Read the model definition and answer for the solid it produces. Units are mm, in the model's axes. A direction names the side the tool comes from. Coordinates: 2 decimals unless noted, no trailing zeros. Loops run counter-clockwise (first coordinate to the right, second up) from the corner with the lowest first, then second, coordinate; pieces in that order, holes last.
from build123d import *

# Parameters (mm, degrees)
BOSS_EXTRUDE1_DEPTH      = 28
BOSS_EXTRUDE1_DEPTH_BACK = 28
CUT_EXTRUDE1_REACH       = 65.151
BOSS_EXTRUDE2_START      = 3
SKETCH5_R                = 1.5000000000000009
BOSS_EXTRUDE2_DEPTH      = 3
CHAMFER1_SIZE            = 0.5
CUT_EXTRUDE2_REACH       = 65.151
SKETCH6_R                = 2.2499999999999987
SKETCH7_R                = 3.7499999999999996
CUT_EXTRUDE3_DEPTH       = 3
CUT_EXTRUDE4_REACH       = 69.039
CUT_EXTRUDE5_DEPTH       = 25.5
FILLET1_R                = 1.5
CUT_EXTRUDE6_DEPTH       = 17.5
CUT_EXTRUDE7_REACH       = 61.059
SKETCH11_R               = 1.5000000000000009
SKETCH11_R_2             = 1.4999999999999987
SKETCH12_W               = 6.9999999999999964
SKETCH12_H               = 5.999999999999993
CUT_EXTRUDE8_DEPTH       = 1


with BuildPart() as part:
    # Sketch3 → Boss-Extrude1 (new, two sides: drawn at the far end of the back side and taken through both)
    with BuildSketch(Plane(origin=(0, 0, 0), x_dir=(0, 0, -1), z_dir=(1, 0, 0)).offset(-BOSS_EXTRUDE1_DEPTH_BACK)):
        Polygon((0, -26.500000000000004), (0, 0), (0, 28.000000000000007), (-7.499999999999999, 28.000000000000007), (-7.5, 48), (29.999999999999996, 48.000000000000014), (30.000000000000004, 13.000000000000009), (3, -26.500000000000004), align=None)
    extrude(amount=BOSS_EXTRUDE1_DEPTH + BOSS_EXTRUDE1_DEPTH_BACK)

    # Cut-Extrude1: up to this plane
    cut_extrude1_end = Plane(origin=(27.999999999999993, 13.000000000000009, -30.000000000000004), z_dir=(0, 0.5643092286475101, 0.8255635011695056))
    # Sketch4 → Cut-Extrude1 (cut, up to the surface)
    with BuildSketch(Plane.XY, mode=Mode.PRIVATE) as cut_extrude1_sk1:
        with BuildLine():
            Line((-22.93301270189222, -21.517949192431118), (-21.387088719442275, -18.84033031018861))
            ThreePointArc((-21.387088719442275, -18.84033031018861), (-20.725616019582173, -17.24339394704681), (-20.5, -15.529670138408827))
            Line((-20.5, -15.529670138408827), (-20.5, -14.499999999999995))
            ThreePointArc((-20.5, -14.499999999999995), (-20.353553390593273, -14.146446609406722), (-20, -13.999999999999995))
            Line((-20, -13.999999999999995), (-10.999999999999998, -13.999999999999995))
            Line((-10.999999999999998, -13.999999999999995), (-11, -1.35e-15))
            ThreePointArc((-11, -1.35e-15), (-1.179e-14, 11), (10.999999999999993, 1.253e-14))
            Line((10.999999999999993, 1.253e-14), (10.999999999999991, -13.999999999999968))
            Line((10.999999999999991, -13.999999999999968), (20.000000000000007, -13.99999999999999))
            ThreePointArc((20.000000000000007, -13.99999999999999), (20.353553390593284, -14.146446609406715), (20.500000000000014, -14.499999999999991))
            Line((20.500000000000014, -14.499999999999991), (20.500000000000014, -15.529670138408822))
            ThreePointArc((20.500000000000014, -15.529670138408822), (20.725616019582187, -17.2433939470468), (21.38708871944229, -18.8403303101886))
            Line((21.38708871944229, -18.8403303101886), (22.933012701892235, -21.51794919243111))
            ThreePointArc((22.933012701892235, -21.51794919243111), (22.98296291314455, -21.897358714982374), (22.750000000000018, -22.200961894323335))
            ThreePointArc((22.750000000000018, -22.200961894323335), (22.012832707939275, -23.304210711669903), (22.43933982822019, -24.560660171779812))
            ThreePointArc((22.43933982822019, -24.560660171779812), (24.587450747697442, -25.99598200005571), (27.12132034355963, -26.499999999999993))
            Line((27.12132034355963, -26.499999999999993), (-27.12132034355962, -26.5))
            ThreePointArc((-27.12132034355962, -26.5), (-24.58745074769743, -25.99598200005572), (-22.43933982822018, -24.56066017177982))
            ThreePointArc((-22.43933982822018, -24.56066017177982), (-22.01283270793929, -23.30421071166992), (-22.750000000000004, -22.200961894323342))
            ThreePointArc((-22.750000000000004, -22.200961894323342), (-22.982962913144537, -21.89735871498238), (-22.93301270189222, -21.517949192431118))
        make_face()
    cut_extrude1_tool1 = split(extrude(cut_extrude1_sk1.sketch, amount=-CUT_EXTRUDE1_REACH, mode=Mode.PRIVATE), bisect_by=cut_extrude1_end, keep=Keep.BOTH, mode=Mode.PRIVATE)
    add(cut_extrude1_tool1.solids().sort_by_distance((0, -11.913251, 0))[0], mode=Mode.SUBTRACT)

    # Sketch5 → Boss-Extrude2 (add)
    with BuildSketch(Plane.XY.offset(BOSS_EXTRUDE2_START)):
        with Locations((23.499999999999996, -23.5)):
            Circle(SKETCH5_R)
        with Locations((-23.500000000000004, -23.5)):
            Circle(SKETCH5_R)
    extrude(amount=-BOSS_EXTRUDE2_DEPTH)

    # Chamfer1
    chamfer1_edges = [part.edges().sort_by_distance(p)[0] for p in [
        (21.999999999999996, -23.5, 3),
        (-25.000000000000004, -23.5, 3),
    ]]
    chamfer(chamfer1_edges, length=CHAMFER1_SIZE)

    # Sketch6 → Cut-Extrude2 (cut, up to next)
    with BuildSketch(Plane.XY, mode=Mode.PRIVATE) as cut_extrude2_sk1:
        with Locations((23.499999999999996, 23.5)):
            Circle(SKETCH6_R)
    cut_extrude2_tool1 = extrude(cut_extrude2_sk1.sketch, amount=-CUT_EXTRUDE2_REACH, mode=Mode.PRIVATE) & part.part
    # Sketch6 → Cut-Extrude2 (cut, up to next)
    with BuildSketch(Plane.XY, mode=Mode.PRIVATE) as cut_extrude2_sk2:
        with Locations((-23.500000000000004, 23.5)):
            Circle(SKETCH6_R)
    cut_extrude2_tool2 = extrude(cut_extrude2_sk2.sketch, amount=-CUT_EXTRUDE2_REACH, mode=Mode.PRIVATE) & part.part
    add(cut_extrude2_tool1.solids().sort_by_distance((23.5, 23.5, 0))[0], mode=Mode.SUBTRACT)
    add(cut_extrude2_tool2.solids().sort_by_distance((-23.5, 23.5, 0))[0], mode=Mode.SUBTRACT)

    # Sketch7 → Cut-Extrude3 (cut)
    with BuildSketch(Plane(origin=(0, 5.95e-15, -30.000000000000007), x_dir=(-1, 0, 0), z_dir=(0, 1.7e-16, -1))):
        with Locations(Location((-23.499999999999996, 23.5, 0), (0, 0, 90))):
            Circle(SKETCH7_R)
        with Locations(Location((23.500000000000004, 23.5, 0), (0, 0, 90))):
            Circle(SKETCH7_R)
    extrude(amount=-CUT_EXTRUDE3_DEPTH, mode=Mode.SUBTRACT)

    # Sketch8 → Cut-Extrude4 (cut, up to next)
    with BuildSketch(Plane(origin=(0, 5.95e-15, -30.000000000000007), x_dir=(-1, 0, 0), z_dir=(0, 2e-16, -1)), mode=Mode.PRIVATE) as cut_extrude4_sk1:
        with BuildLine():
            Line((-10.749999999999991, 40.000000000000014), (-10.749999999999993, 48.00000000000001))
            Line((-10.749999999999993, 48.00000000000001), (10.749999999999995, 48.00000000000001))
            Line((10.749999999999995, 48.00000000000001), (10.750000000000004, 40.000000000000014))
            ThreePointArc((10.750000000000004, 40.000000000000014), (4.96e-15, 29.250000000000014), (-10.749999999999991, 40.000000000000014))
        make_face()
    cut_extrude4_tool1 = extrude(cut_extrude4_sk1.sketch, amount=-CUT_EXTRUDE4_REACH, mode=Mode.PRIVATE) & part.part
    add(cut_extrude4_tool1.solids().sort_by_distance((0, 39.603429, -30))[0], mode=Mode.SUBTRACT)

    # Sketch9 → Cut-Extrude5 (cut)
    with BuildSketch(Plane(origin=(0, 5.95e-15, -30.000000000000007), x_dir=(-1, 0, 0), z_dir=(0, 2e-16, -1))):
        with BuildLine():
            Line((3.5000000000000053, 27.700862818523312), (15.002567384846198, 32.500000000000014))
            ThreePointArc((15.002567384846198, 32.500000000000014), (19.704089145058386, 37.826997771928276), (18.41995596409805, 44.815002787484154))
            ThreePointArc((18.41995596409805, 44.815002787484154), (18.246442865607545, 46.902775048106754), (20.03109891440682, 48.00000000000001))
            Line((20.03109891440682, 48.00000000000001), (-20.031098914406805, 48.000000000000014))
            ThreePointArc((-20.031098914406805, 48.000000000000014), (-18.24644286560753, 46.90277504810676), (-18.419955964098037, 44.81500278748416))
            ThreePointArc((-18.419955964098037, 44.81500278748416), (-19.70408914505838, 37.82699777192828), (-15.002567384846188, 32.500000000000014))
            Line((-15.002567384846188, 32.500000000000014), (-3.4999999999999947, 27.700862818523312))
            ThreePointArc((-3.4999999999999947, 27.700862818523312), (4.59e-15, 27.00000000000002), (3.5000000000000053, 27.700862818523312))
        make_face()
    extrude(amount=-CUT_EXTRUDE5_DEPTH, mode=Mode.SUBTRACT)

    # Fillet1
    fillet1_edges = [part.edges().sort_by_distance(p)[0] for p in [
        (10.749999999999993, 48.00000000000001, 1.5000000000000036),
        (-10.749999999999995, 48.00000000000001, 1.5000000000000036),
        (-10.75, 44.000000000000014, -4.499999999999998),
        (-15.390549457203406, 48.00000000000001, -4.499999999999997),
        (15.390549457203399, 48.000000000000014, -4.499999999999997),
        (-3.8e-15, 29.250000000000014, -4.500000000000002),
        (10.749999999999993, 44.000000000000014, -4.499999999999999),
    ]]
    fillet(fillet1_edges, radius=FILLET1_R)

    # Sketch10 → Cut-Extrude6 (cut)
    with BuildSketch(Plane(origin=(0, 5.95e-15, -30.000000000000007), x_dir=(-1, 0, 0), z_dir=(0, 2e-16, -1))):
        with BuildLine():
            Line((17.312884960931758, 32.96263305373123), (28.000000000000007, 32.962633053731224))
            Line((28.000000000000007, 32.962633053731224), (28.000000000000007, 48.00000000000001))
            Line((28.000000000000007, 48.00000000000001), (20.03109891440682, 48.00000000000001))
            ThreePointArc((20.03109891440682, 48.00000000000001), (18.24644286560754, 46.902775048106754), (18.41995596409805, 44.815002787484154))
            ThreePointArc((18.41995596409805, 44.815002787484154), (19.704089145058383, 37.826997771928276), (15.002567384846198, 32.500000000000014))
            ThreePointArc((15.002567384846198, 32.500000000000014), (16.1347936396864, 32.84583803391052), (17.312884960931758, 32.96263305373123))
        make_face()
        with BuildLine():
            Line((-17.312884960931758, 32.96263305373123), (-28.000000000000007, 32.962633053731224))
            Line((-28.000000000000007, 32.962633053731224), (-28.000000000000007, 48.00000000000001))
            Line((-28.000000000000007, 48.00000000000001), (-20.03109891440682, 48.00000000000001))
            ThreePointArc((-20.03109891440682, 48.00000000000001), (-18.24644286560754, 46.902775048106754), (-18.41995596409805, 44.815002787484154))
            ThreePointArc((-18.41995596409805, 44.815002787484154), (-19.704089145058383, 37.826997771928276), (-15.002567384846198, 32.500000000000014))
            ThreePointArc((-15.002567384846198, 32.500000000000014), (-16.1347936396864, 32.84583803391052), (-17.312884960931758, 32.96263305373123))
        make_face()
    extrude(amount=-CUT_EXTRUDE6_DEPTH, mode=Mode.SUBTRACT)

    # Sketch11 → Cut-Extrude7 (cut, up to next)
    with BuildSketch(Plane(origin=(0, 5.4e-16, -12.500000000000002), x_dir=(-1, 0, 0), z_dir=(0, 4e-17, -1)), mode=Mode.PRIVATE) as cut_extrude7_sk1:
        with Locations(Location((24.000000000000007, 40.00000000000002, 0), (0, 0, 90))):
            Circle(SKETCH11_R)
    cut_extrude7_tool1 = extrude(cut_extrude7_sk1.sketch, amount=-CUT_EXTRUDE7_REACH, mode=Mode.PRIVATE) & part.part
    # Sketch11 → Cut-Extrude7 (cut, up to next)
    with BuildSketch(Plane(origin=(0, 5.4e-16, -12.500000000000002), x_dir=(-1, 0, 0), z_dir=(0, 4e-17, -1)), mode=Mode.PRIVATE) as cut_extrude7_sk2:
        with Locations(Location((-24, 39.99999999999999, 0), (0, 0, 90))):
            Circle(SKETCH11_R_2)
    cut_extrude7_tool2 = extrude(cut_extrude7_sk2.sketch, amount=-CUT_EXTRUDE7_REACH, mode=Mode.PRIVATE) & part.part
    add(cut_extrude7_tool1.solids().sort_by_distance((-24, 40, -12.5))[0], mode=Mode.SUBTRACT)
    add(cut_extrude7_tool2.solids().sort_by_distance((24, 40, -12.5))[0], mode=Mode.SUBTRACT)

    # Sketch12 → Cut-Extrude8 (cut, symmetric)
    with BuildSketch(Plane(origin=(0, 1.1e-16, -2.5000000000000027), x_dir=(-1, 0, 0), z_dir=(0, 4e-17, -1))):
        with Locations((24.500000000000007, 40.00000000000003)):
            Rectangle(SKETCH12_W, SKETCH12_H)
        Polygon((-28.000000000000007, 43.000000000000014), (-28.000000000000007, 37.00000000000002), (-21.00000000000001, 37.00000000000003), (-21.00000000000001, 43.000000000000014), align=None)
    extrude(amount=CUT_EXTRUDE8_DEPTH, both=True, mode=Mode.SUBTRACT)


solid = part.part
Q1. Which of the six approach directions +Z, -Z, +X, -X, +Y, -Y give full straight-line access (tool end or side, diameter ignored) to faces 1 (the face through (-26, 40, -3.5)), 2 (the face through (-24.6, -26, -1.7)), 3 (the face through (16.119, 32.843, -21.372)), 4 (the face through (26, 40, -1.5))?
Findings below:
face 1: -X
face 2: +Z, -Z, -Y
face 3: -Z, +Y
face 4: +X
Q2. A cutting plane is placed at D-D (y = -20.5). Give the vertices of the cut face in (x, z).
Findings below:
outline: (-28, -7.1) - (-22.35, -7.1) - (-22.35, 0) - (-28, 0) - close; (22.35, -7.1) - (28, -7.1) - (28, 0) - (22.35, 0) - close
Q3. A cutting plane is placed at A-A (z = 1). Give the vertices of the cut face in (x, y).
Findings below:
outline: (-28, 28) - (28, 28) - (28, 48) - (12.25, 48) arc R1.5 ccw to (10.75, 46.5) - (10.75, 40) arc R10.75 cw to (-10.75, 40) - (-10.75, 46.5) arc R1.5 ccw to (-12.25, 48) - (-28, 48) - close; circle Ø3 at (-23.5, -23.5); circle Ø3 at (23.5, -23.5); hole circle Ø3 at (-24, 40); hole circle Ø3 at (24, 40)
Q4. A cutting plane is placed at C-C (x = 0). Give the vertices of the cut face in (y, z).
Findings below:
outline: (11, -28.63) - (13, -30) - (27, -30) - (27, -4.5) - (27.75, -4.5) arc R1.5 ccw to (29.25, -3) - (29.25, 7.5) - (28, 7.5) - (28, 0) - (11, 0) - close
Q5. Straight lines are drawn through the part: probe 1 along X at (y, z) = (23.5, -28.7); probe 2 along X at (y, z) = (-11, -7.5); probe 3 along Y at (x, z) = (-24, -9). For each, find the intervals that lie inside material, in ascending order.
Findings below:
probe 1: x = -28 to -27.25, -19.75 to 19.75, 27.25 to 28
probe 2: x = -28 to -11, 11 to 28
probe 3: y = -17.72 to 21.31, 25.69 to 38.5, 41.5 to 48
Q6. Determine the mould class of faces 5 (the face through (-21, 40, -2)), 6 (the face through (25.01, 38.89, -8.06)), 7 (the face through (0, 23, -30)) for opening direction X: +X half, -X half, draft (parallel to the pull), parting line (faces both ways), or undercut.
Findings below:
face 5: -X half
face 6: undercut
face 7: draft
Q7. A cutting plane is placed at B-B (y = -3). Give the vertices of the cut face in (x, z), then the cut area to 3 significant figures.
Findings below:
outline: (-28, -19.06) - (-11, -19.06) - (-11, 0) - (-28, 0) - close; (11, -19.06) - (28, -19.06) - (28, 0) - (11, 0) - close
area: 648 mm2
Q8. Flat-ended cylindrical pins translate along their axes: pin 1 Ø12 at (x, y) = (-13, -19) entering from -Z; pin 2 Ø3 at (x, z) = (11, -21) entering from -Y; pin 3 Ø1.6 at (x, y) = (-23, -23) entering from +Z. Find the tip coordinate at first contact, or state that the pin passes through.
Findings below:
pin 1: stops at z = -12.23
pin 2: stops at y = -2.36
pin 3: stops at z = 3
